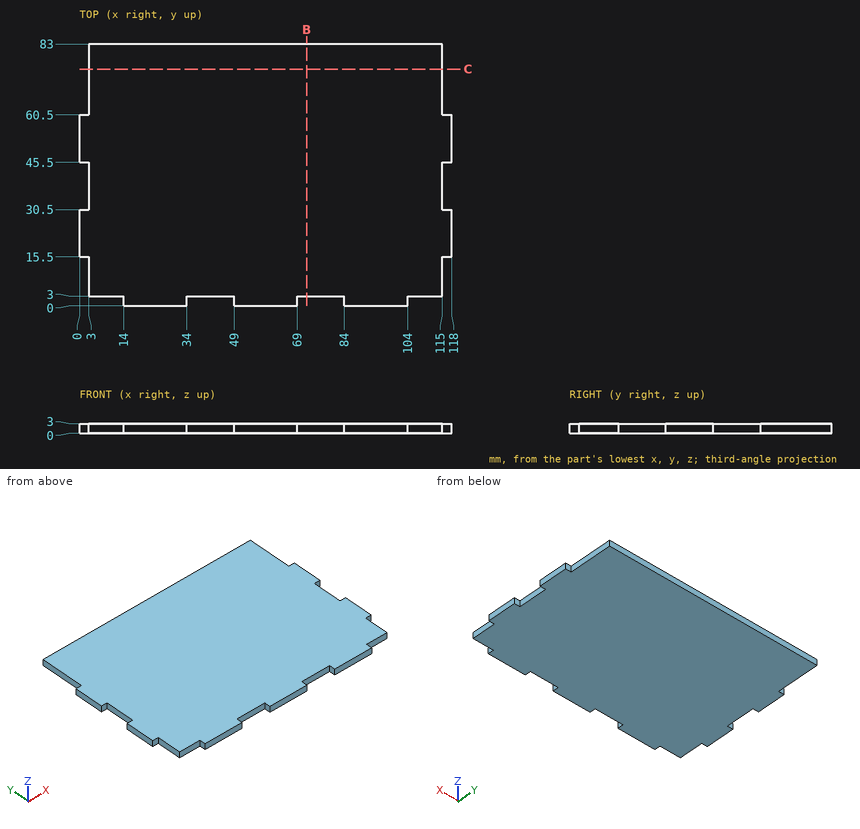
Geometry check sheet. Reference: drawing and pictorial views, mm from the part's lowest x, y, z. Round coordinates to 2 decimals unless told otherwise and drop trailing zeros. Loops run counter-clockwise (first coordinate to the right, second up) from the corner with the lowest first, then second, coordinate; pieces in that order, holes last. Notation, with made-up numbers: M 22,81.5 L 29,81.5 A20 cw 29,111.5 Z; hole C 25.5,29 d11. An arc over 180 degrees is marked long. Return JSON: item names as keys, results as strings. Group by question number.
(1) Scan lines: line 1 along Y through (x, z) = (38, 2.1); line 2 along X through (y, z) = (77, 0.9). Record each from-to range of solid material in increasing order. Write a range as [from, to].
(2) Section check C-C, the plane y = 75. Enter the section's corners in (x, z).
(3) Go/stop test with flat-tipped pins: pin 1 (1.5 mm diameter, centred on y = 1.5, z = 1, fed in from +X); pin 2 (0.9 mm diameter, centred on x = 2, z = 1.5, fed in from -Y); pin 3 (0.9 mm diameter, centred on x = 1.5, z = 1, fed in from +Y). Record where each tip stops, or that it passes through.
(4) Section check B-B, the plane x = 72. Enter the section's corners in (y, z).
Data:
{
 "1": {"line 1": "[3, 83]", "line 2": "[3, 115]"},
 "2": {"outline": "M 3,0 L 115,0 L 115,3 L 3,3 Z"},
 "3": {"pin 1": "x = 104", "pin 2": "y = 15.5", "pin 3": "y = 60.5"},
 "4": {"outline": "M 3,0 L 83,0 L 83,3 L 3,3 Z"}
}
